from build123d import *

# Parameters (mm, degrees)
F1_DEPTH = 50.8
F2_W     = 25.4
F2_H     = 25.4
F3_DEPTH = 11.5072
F4_R     = 3.2131
F5_DEPTH = 101.601
F6_R     = 3.175
F7_DEPTH = 2.54


with BuildPart() as f1:
    # F0 (on Top) → F1 (new body, symmetric)
    with BuildSketch(Plane.XY):
        with BuildLine():
            ThreePointArc((-4.772227, 3.2131), (2.703042, -5.078555), (0, 5.7531))
            Line((0, 5.7531), (-11.1379, 5.7531))
            Line((-11.1379, 5.7531), (-11.1379, 16.8021))
            Line((-11.1379, 16.8021), (11.7221, 16.8021))
            Line((11.7221, 16.8021), (11.7221, 19.3421))
            Line((11.7221, 19.3421), (-13.6779, 19.3421))
            Line((-13.6779, 19.3421), (-13.6779, 3.2131))
            Line((-13.6779, 3.2131), (-4.772227, 3.2131))
        make_face()
    extrude(amount=F1_DEPTH, both=True)

    # F2 (on face) → F3 (cut, through all)
    with BuildSketch(Plane(origin=(0, 5.7531, 0), x_dir=(-1, 0, 0), z_dir=(0, 1, 0))):
        with Locations((-5.3721, 25.4)):
            Rectangle(F2_W, F2_H)
        with Locations((-5.3721, -25.4)):
            Rectangle(F2_W, F2_H)
    extrude(amount=-F3_DEPTH, mode=Mode.SUBTRACT)

    # F4 (on face) → F5 (cut, through all)
    with BuildSketch(Plane.XY.offset(50.8)):
        Circle(F4_R)
    extrude(amount=-F5_DEPTH, mode=Mode.SUBTRACT)

    # F6 (on face) → F7 (cut, through all)
    with BuildSketch(Plane(origin=(0, 19.3421, 0), x_dir=(-1, 0, 0), z_dir=(0, 1, 0))):
        with Locations((-2.8321, 25.4)):
            Circle(F6_R)
        with Locations((-2.8321, -25.4)):
            Circle(F6_R)
    extrude(amount=-F7_DEPTH, mode=Mode.SUBTRACT)


solid = f1.part
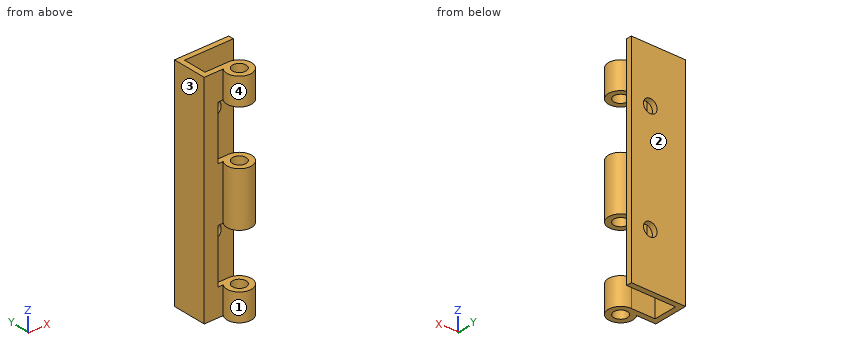
For this review, take the finished solid that the model builds, in its own axes (mm). Face numbers are marked on the shaded views. Round coordinates to 2 decimals unless told otherwise and drop trailing zeros. Write each loop counter-clockwise with the first axis right and the second up, starting at its lowest first coordinate (ties: lowest second). Pieces come first, ordered by that corner, then holes. Notation, with made-up numbers: M 61,-8 L 95,-8 A16 cw 95,-3 Z; hole C 7,-38.5 d4. An arc over 180 degrees is marked long. Write item = value, one per line. Start each with the question number.
(1) We need section C-C (x = -10). Give the boundary of the cut face in (y, z).
(2) Clearance check with flat-ended pins moving along their axes: pin 1 Ø5.5 at (y, z) = (10, 8.5) entering from +X; pin 2 Ø1.5 at (x, z) = (7.5, -28) entering from -Y; pin 3 Ø4 at (x, y) = (0, 0) entering from -Z; pin 4 Ø7 at (x, z) = (-7.5, 21.5) entering from -Y. State where each tip first meets the part, or that it passes through.
(3) For line 1 along Z through (x, y) = (-0.75, 4); line 2 along Z through (x, y) = (5.5, 17.25); line 3 along X through (y, z) = (-0.25, 42), list the stretches that pass through material, from the lowest coordinate up.
(4) We need section D-D (z = 10). Give the boundary of the cut face in (x, y).
(5) We need section A-A (z = 25.4). Give the boundary of the cut face in (x, y).
(6) The part is to be moulded in two halves that separate along Y. For the marked faces 1, 2, 3 and 4, say which applies: +Y half, -Y half, draft (parallel to the pull), parting line (faces both ways), or undercut.
(7) We need section B-B (y = 0). Give the boundary of the cut face in (x, z).
Results found:
q1.outline = M 3.21,-50.8 L 5.75,-50.8 L 5.75,50.8 L 3.21,50.8 Z; M 16.8,-50.8 L 19.34,-50.8 L 19.34,50.8 L 16.8,50.8 Z
q2.pin_1 = -11.14
q2.pin_2 = 16.8
q2.pin_3 = through
q2.pin_4 = 3.21
q3.line_1 = -50.8 to -38.1, -12.7 to 12.7, 38.1 to 50.8
q3.line_2 = -50.8 to -27.12, -23.68 to 23.68, 27.12 to 50.8
q3.line_3 = -5.75 to -3.2, 3.2 to 5.75
q4.outline = M -13.68,3.21 L -4.77,3.21 A5.75 ccw long 0,5.75 L -11.14,5.75 L -11.14,16.8 L 11.72,16.8 L 11.72,19.34 L -13.68,19.34 Z; hole C 0,0 d6.43
q5.outline = M -13.68,3.21 L -7.33,3.21 L -7.33,5.75 L -11.14,5.75 L -11.14,16.8 L -0.34,16.8 L -0.34,19.34 L -13.68,19.34 Z; M 6.01,16.8 L 11.72,16.8 L 11.72,19.34 L 6.01,19.34 Z
q6.face_1 = undercut
q6.face_2 = +Y half
q6.face_3 = draft
q6.face_4 = undercut
q7.outline = M -5.75,-50.8 L -3.21,-50.8 L -3.21,-38.1 L -5.75,-38.1 Z; M -5.75,-12.7 L -3.21,-12.7 L -3.21,12.7 L -5.75,12.7 Z; M -5.75,38.1 L -3.21,38.1 L -3.21,50.8 L -5.75,50.8 Z; M 3.21,-50.8 L 5.75,-50.8 L 5.75,-38.1 L 3.21,-38.1 Z; M 3.21,-12.7 L 5.75,-12.7 L 5.75,12.7 L 3.21,12.7 Z; M 3.21,38.1 L 5.75,38.1 L 5.75,50.8 L 3.21,50.8 Z
